```python
from build123d import *
from build123d.topology import SkipClean

# Parameters (mm, degrees)
BOSS_EXTRUDE1_START   = 2
BOSS_EXTRUDE1_DEPTH   = 2
MIRROR_START          = 2
MIRROR_2_COPY_1_DEPTH = 2
MIRROR_2_COPY_2_DEPTH = 2


with BuildPart() as part:
    # Sketch2 → Revolve1 (revolve)
    with BuildSketch(Plane.XY, mode=Mode.PRIVATE) as revolve1_sk:
        Polygon((2.475, 2), (2.475, 1.2), (1.245, 1.2), (1.245, 0.45), (2.375, 0.45), (2.375, -2), (3.535, -2), (3.535, 2), align=None)
    revolve(revolve1_sk.sketch.rotate(Axis((0, 55, 0), (0, -1, 0)), 90), axis=Axis((0, 55, 0), (0, -1, 0)))

    # Sketch3 → Boss-Extrude1 (add)
    with BuildSketch(Plane(origin=(0, 0, 0), x_dir=(1, 0, 0), z_dir=(0, 1, 0)).offset(BOSS_EXTRUDE1_START)):
        with BuildLine():
            ThreePointArc((3.535, 0), (3.180996027, -1.541910917), (2.189885842, -2.775))
            Line((2.189885842, -2.775), (14.232465575, -1.773881029))
            ThreePointArc((14.232465575, -1.773881029), (13.044016702, -1.443867644), (12.3554, -0.420575606))
            ThreePointArc((12.3554, -0.420575606), (11.845417029, -0.438862165), (11.585, 0))
            Line((11.585, 0), (10.585, 0))
            ThreePointArc((10.585, 0), (10.085, -0.5), (9.585, 0))
            Line((9.585, 0), (8.585, 0))
            ThreePointArc((8.585, 0), (8.085, -0.5), (7.585, 0))
            Line((7.585, 0), (6.585, 0))
            ThreePointArc((6.585, 0), (6.085, -0.5), (5.585, 0))
            Line((5.585, 0), (4.585, 0))
            ThreePointArc((4.585, 0), (4.085, -0.5), (3.585, 0))
            Line((3.585, 0), (3.535, 0))
        make_face()
        with BuildLine():
            ThreePointArc((12.3554, -0.420575606), (13.044016702, -1.443867644), (14.232465575, -1.773881029))
            ThreePointArc((14.232465575, -1.773881029), (15.394749733, -1.205386095), (15.865, 0))
            Line((15.865, 0), (14.585, 0))
            ThreePointArc((14.585, 0), (14.085, -0.5), (13.585, 0))
            Line((13.585, 0), (12.585, 0))
            ThreePointArc((12.585, 0), (12.523862165, -0.239582971), (12.3554, -0.420575606))
        make_face()
    boss_extrude1 = extrude(amount=-BOSS_EXTRUDE1_DEPTH)

    # Mirror1: Boss-Extrude1 across plane
    with SkipClean():  # the faces are left unmerged after this step: merging them gives an invalid solid
        add(boss_extrude1.mirror(Plane(origin=(0, 15.95383002, 0), x_dir=(1, 0, 0), z_dir=(0, 0, -1))))

    # 镜向1: Boss-Extrude1 across plane
    with SkipClean():  # the faces are left unmerged after this step: merging them gives an invalid solid
        add(boss_extrude1.mirror(Plane(origin=(0, 0, 0), x_dir=(0, 0, 1), z_dir=(1, 0, 0))))

    # 镜向2 copy 1 sketch → 镜向2 copy 1 (add)
    with SkipClean():  # the faces are left unmerged after this step: merging them gives an invalid solid
        with BuildSketch(Plane(origin=(0, 0, 0), x_dir=(-1, 0, 0), z_dir=(0, 1, 0)).offset(MIRROR_START)):
            with BuildLine():
                ThreePointArc((3.535, 0), (3.180996027, -1.541910917), (2.189885842, -2.775))
                Line((2.189885842, -2.775), (14.232465575, -1.773881029))
                ThreePointArc((14.232465575, -1.773881029), (13.044016702, -1.443867644), (12.3554, -0.420575606))
                ThreePointArc((12.3554, -0.420575606), (11.845417029, -0.438862165), (11.585, 0))
                Line((11.585, 0), (10.585, 0))
                ThreePointArc((10.585, 0), (10.085, -0.5), (9.585, 0))
                Line((9.585, 0), (8.585, 0))
                ThreePointArc((8.585, 0), (8.085, -0.5), (7.585, 0))
                Line((7.585, 0), (6.585, 0))
                ThreePointArc((6.585, 0), (6.085, -0.5), (5.585, 0))
                Line((5.585, 0), (4.585, 0))
                ThreePointArc((4.585, 0), (4.085, -0.5), (3.585, 0))
                Line((3.585, 0), (3.535, 0))
            make_face()
            with BuildLine():
                ThreePointArc((12.3554, -0.420575606), (13.044016702, -1.443867644), (14.232465575, -1.773881029))
                ThreePointArc((14.232465575, -1.773881029), (15.394749733, -1.205386095), (15.865, 0))
                Line((15.865, 0), (14.585, 0))
                ThreePointArc((14.585, 0), (14.085, -0.5), (13.585, 0))
                Line((13.585, 0), (12.585, 0))
                ThreePointArc((12.585, 0), (12.523862165, -0.239582971), (12.3554, -0.420575606))
            make_face()
        extrude(amount=-MIRROR_2_COPY_1_DEPTH)

    # 镜向2 copy 2 sketch → 镜向2 copy 2 (add)
    with SkipClean():  # the faces are left unmerged after this step: merging them gives an invalid solid
        with BuildSketch(Plane(origin=(0, 0, 0), x_dir=(1, 0, 0), z_dir=(0, 1, 0)).offset(MIRROR_START)):
            with BuildLine():
                ThreePointArc((3.535, 0), (3.180996027, 1.541910917), (2.189885842, 2.775))
                Line((2.189885842, 2.775), (14.232465575, 1.773881029))
                ThreePointArc((14.232465575, 1.773881029), (13.044016702, 1.443867644), (12.3554, 0.420575606))
                ThreePointArc((12.3554, 0.420575606), (11.845417029, 0.438862165), (11.585, 0))
                Line((11.585, 0), (10.585, 0))
                ThreePointArc((10.585, 0), (10.085, 0.5), (9.585, 0))
                Line((9.585, 0), (8.585, 0))
                ThreePointArc((8.585, 0), (8.085, 0.5), (7.585, 0))
                Line((7.585, 0), (6.585, 0))
                ThreePointArc((6.585, 0), (6.085, 0.5), (5.585, 0))
                Line((5.585, 0), (4.585, 0))
                ThreePointArc((4.585, 0), (4.085, 0.5), (3.585, 0))
                Line((3.585, 0), (3.535, 0))
            make_face()
            with BuildLine():
                ThreePointArc((12.3554, 0.420575606), (13.044016702, 1.443867644), (14.232465575, 1.773881029))
                ThreePointArc((14.232465575, 1.773881029), (15.394749733, 1.205386095), (15.865, 0))
                Line((15.865, 0), (14.585, 0))
                ThreePointArc((14.585, 0), (14.085, 0.5), (13.585, 0))
                Line((13.585, 0), (12.585, 0))
                ThreePointArc((12.585, 0), (12.523862165, 0.239582971), (12.3554, 0.420575606))
            make_face()
        extrude(amount=-MIRROR_2_COPY_2_DEPTH)


solid = part.part
```
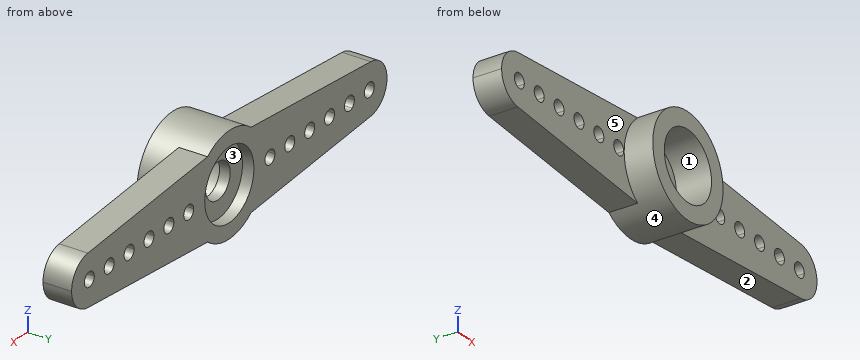
Can you work these out from the model? Positions are in its coordinate system, mm. Face numbers are marked on the shaded views. A direction names the side the tool comes from. Round coordinates to 2 decimals unless told otherwise and drop trailing zeros. Loops run counter-clockwise (first coordinate to the right, second up) from the corner with the lowest first, then second, coordinate; pieces in that order, holes last.
Item 1: If we mould it in two halves opening along X, with no side actions, what happens to the marked faces 3, 4 and 5? For each: +X half, -X half, draft (parallel to the pull), parting line (faces both ways), or undercut.
Item 2: Suppose I cut it at B-B, the plane x = 4. Write out the boundary of the cut face in (y, z).
Item 3: Which directions (+Z, -Z, +X, -X, +Y, -Y) give clear straight access to the entire face, cutting with the end or side of a thin tool? Please do the marked faces 1 and 2.
Item 4: Will these pins go through, and if not, where does the flat tip stop? pin 1 Ø2.5 at (x, z) = (-0.5, 0.5) entering from -Y; pin 2 Ø1.5 at (x, z) = (0, 0) entering from +Y; pin 3 Ø2 at (y, z) = (-0.5, -1.5) entering from +X; pin 4 Ø1 at (x, y) = (-3.5, 0) entering from -Z.
Item 5: Please list where these lines run through material, in increasing order: L1, parallel to X at y = -1.05, z = 0 (3 decimals); L2, parallel to Y at x = 10.5, z = -0.5; L3, parallel to Z at x = -11.5, y = 0.25.
Item 6: Suppose I cut it at A-A, the plane x = 0. Write out the boundary of the cut face in (y, z) (3 decimals), then the cut area to 3 significant figures.
Reported:
1. face 3: undercut
1. face 4: parting line
1. face 5: draft
2. outline: (0, -2.62) - (2, -2.62) - (2, -0.49) - (0, -0.49) - close; (0, 0.49) - (2, 0.49) - (2, 2.62) - (0, 2.62) - close
3. face 1: -Y
3. face 2: -Z, +X, +Y, -Y
4. pin 1: stops at y = 0.45
4. pin 2: passes through
4. pin 3: stops at x = 15.75
4. pin 4: stops at z = -2.71
5. L1: x = -3.535 to -2.375, 2.375 to 3.535
5. L2: y = 0 to 2
5. L3: z = -2 to 2
6. outline: (-2, -3.535) - (2, -3.535) - (2, -2.475) - (1.2, -2.475) - (1.2, -1.245) - (0.45, -1.245) - (0.45, -2.375) - (-2, -2.375) - close; (-2, 2.375) - (0.45, 2.375) - (0.45, 1.245) - (1.2, 1.245) - (1.2, 2.475) - (2, 2.475) - (2, 3.535) - (-2, 3.535) - close
6. area: 10.8 mm2
